Autodesk Inventor part; units mm, degrees
ref_plane "YZ Plane" through (0, 0, 0) normal (1, 0, 0) x (0, 1, 0)
ref_plane "XZ Plane" through (0, 0, 0) normal (0, 1, 0) x (-1, 0, 0)
ref_plane "XY Plane" through (0, 0, 0) normal (0, 0, 1) x (1, 0, 0)
sketch "Эскиз1" plane through (0, 0, 0) normal (0, 0, 1) x (1, 0, 0)
  line L0 (-11.75, -4.5) -> (11.75, -4.5)
  line L1 (11.75, -4.5) -> (11.75, 4.5)
  line L2 (11.75, 4.5) -> (-11.75, 4.5)
  line L3 (-11.75, 4.5) -> (-11.75, -4.5)
  line L4 (-11.75, -4.5) -> (11.75, 4.5) construction
  line L5 (11.75, -4.5) -> (-11.75, 4.5) construction
  point P0 (0, 0)
  dimension "d0" = 23.5
  dimension "d1" = 9
extrude "Выдавливание1" add sketch "Эскиз1" along normal mid plane 17
sketch "Эскиз2" plane through (0, 0, 0) normal (0, 1, 0) x (-1, 0, 0)
  line L0 (14.5, -3.1) -> (-14.5, -3.1)
  line L1 (-14.5, -3.1) -> (-14.5, -7.1)
  line L2 (-14.5, -7.1) -> (14.5, -7.1)
  line L3 (14.5, -7.1) -> (14.5, -3.1)
  line L4 (-11.75, 8.5) -> (11.75, 8.5)
  line L5 (0, 8.5) -> (0, -8.5)
  line L6 (11.75, -8.5) -> (-11.75, -8.5)
  line L7 (14.5, -5.1) -> (-14.5, -5.1)
  line L8 (13.25, -5.1) -> (-13.25, -5.1)
  circle A0 centre (13.25, -5.1) radius 0.75
  circle A1 centre (-13.25, -5.1) radius 0.75
  point P0 (0, 0)
  point P1 (0, -7.1)
  point P2 (0, -5.1)
  dimension "d4" = 29
  dimension "d5" = 4
  dimension "d6" = 26.5
  dimension "d7" = 1.5
  dimension "d8" = 1.5
  dimension "d9" = 3.4
extrude "Выдавливание2" add sketch "Эскиз2" along normal mid plane 0.95 contours L3 L7 A0 L5 L0 | L5 L7 A1 L1 L0 | L3 L2 L5 L7 A0 | L5 L2 L1 L7 A1
fillet "Сопряжение1" radius 4.5 4 edges at (-11.75, -4.5, 0) (-11.75, 4.5, 0) (11.75, 4.5, 0) (11.75, -4.5, 0)
sketch "Эскиз3" plane through (0, 0, 8.5) normal (0, 0, 1) x (1, 0, 0)
  arc A0 (7.25, -4.5) -> (7.25, 4.5) centre (7.25, 0) ccw
  circle A1 centre (7.25, 0) radius 3.5
  point P0 (0, 0)
  dimension "d13" = 7
extrude "Выдавливание3" add sketch "Эскиз3" along normal blind 3.5
sketch "Эскиз4" plane through (-7.25, 4.5, -8.5) normal (0, 1, 0) x (1, 0, 0)
  line L0 (0, -17) -> (-4.5, -17)
  line L1 (-4.5, -17) -> (-4.5, -15.5)
  line L2 (-4.5, 0) -> (-4.5, -17)
  line L3 (-4.5, -17) -> (-0.5, -17)
  line L4 (-0.5, -17) -> (-4.5, -15.5)
  point P0 (7.25, -8.5)
  dimension "d16" = 1.5
  dimension "d17" = 4
extrude "Выдавливание4" cut sketch "Эскиз4" against normal blind 20
sketch "Эскиз5" plane through (0, 0, -8.5) normal (0, 0, -1) x (-1, 0, 0)
  line L0 (14.5, -0.475) -> (14.5, 0.475)
  line L1 (14.5, 0) -> (-14.5, 0)
  line L2 (-14.5, -0.475) -> (-14.5, 0.475)
  circle A0 centre (5.95, 0) radius 4
  line L3 (12.5, 0.475) -> (12.5, -0.475)
  line L4 (12.5, 0) -> (14, 0)
  line L5 (14, 0.475) -> (14, -0.475)
  line L6 (13.25, 0) -> (5.95, 0)
  point P0 (0, 0)
  dimension "d20" = 8
  dimension "d21" = 7.3
extrude "Выдавливание5" add sketch "Эскиз5" along normal blind 0.8
sketch "Эскиз6" plane through (-5.95, 0, -9.3) normal (0, 0, -1) x (-1, 0, 0)
  circle A0 centre (0, 0) radius 1.925
  point P0 (-5.95, 0)
  dimension "d24" = 3.85
extrude "Выдавливание6" add sketch "Эскиз6" along normal blind 3
chamfer "Фаска1" distance 0.3 angle 45 1 edges at (-4.025, 0, -12.3)
sketch "Эскиз7" plane through (0, 0, -8.5) normal (0, 0, -1) x (-1, 0, 0)
  circle A0 centre (5.95, 0) radius 4
  arc A1 (-7.25, 4.5) -> (-7.25, -4.5) centre (-7.25, 0) ccw
  line L0 (-7.25, -4.5) -> (7.25, -4.5)
  arc A2 (7.25, -4.5) -> (7.25, 4.5) centre (7.25, 0) ccw
  line L1 (7.25, 4.5) -> (-7.25, 4.5)
  line L2 (7.25, -4.5) -> (-7.25, -4.5)
  line L3 (-7.25, -4.5) -> (-7.25, 4.5)
  line L4 (-7.25, 4.5) -> (7.25, 4.5)
  line L5 (7.25, 4.5) -> (7.25, -4.5)
  circle A3 centre (5.95, 0) radius 1.925
  circle A4 centre (5.95, 0) radius 4
  circle A5 centre (5.95, 0) radius 1.625
  point P0 (0, 0)
properties part number "OCS-D008 B"
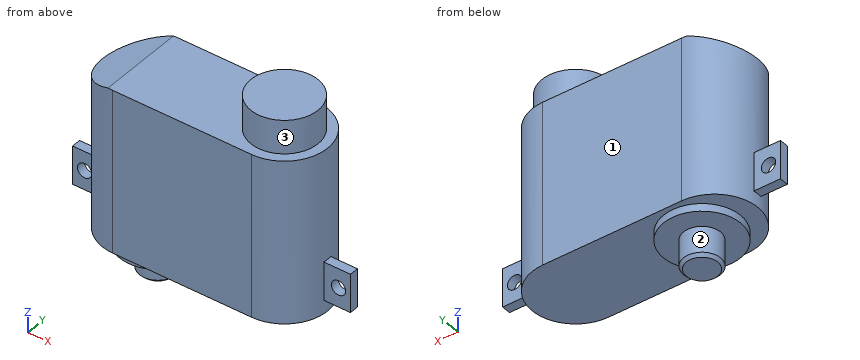
Input: part model. Units: mm. Frame: model coordinates. Face numbers are marked on the shaded views. A direction names the side the tool comes from. Give positions to 0.01 mm unless a question says otherwise; leave off trailing zeros. Order: outer loops, then holes, each group sorted by start corner. A loop starts at its lowest first (then second) coordinate and runs counter-clockwise, first axis right, second up. Notation, with made-up numbers: M 15.25,30 L 28.25,30 A22 ccw 28.25,60 Z; hole C 86.25,2 d11. An arc over 180 degrees is marked long. Return JSON: item names as keys, results as strings.
1) Access query for the marked faces 1, 2 and 3. Directions: +Z, -Z, +X, -X, +Y, -Y. A direction counts if a zero-diameter tool reaches every point of the face in a straight line with its end or side. Return the directions, or none.
Taken from the geometry:
{"face 1": "+Z, -Z, +X, -X, +Y", "face 2": "-Z", "face 3": "+Z"}
2) Line query: L1, parallel to X at y = -0.2, z = -5.1; L2, parallel to Z at x = -13.25, y = 0.1; L3, parallel to Z at x = 5.75, y = -2.75. Output: solid intervals per line, ascending. Write a range as [from, to].
Taken from the geometry:
{"L1": "x = [-14.5, -14], [-12.5, 12.5], [14, 14.5]", "L2": "z = [-7.1, -5.85], [-4.35, -3.1]", "L3": "z = [-8.5, 12]"}
3) Section query B-B on x = -5.95. Output: boundary loops of the cut face in (y, z) (3 decimals), and give its area (3 significant figures).
Taken from the geometry:
{"outline": "M -4.5,-8.5 L -4,-8.5 L -4,-9.3 L -1.925,-9.3 L -1.925,-12 L -1.625,-12.3 L 1.625,-12.3 L 1.925,-12 L 1.925,-9.3 L 4,-9.3 L 4,-8.5 L 4.5,-8.5 L 4.5,8.5 L -4.5,8.5 Z", "area": "171 mm2"}
4) Section query A-A on z = -5.1. Output: boundary loops of the cut face in (x, y) (3 decimals), and give its area (3 significant figures).
Taken from the geometry:
{"outline": "M -14.5,-0.475 L -14,-0.475 L -14,0.475 L -14.5,0.475 Z; M -12.5,-0.475 L -11.725,-0.475 A4.5 ccw -7.25,-4.5 L 7.25,-4.5 A4.5 ccw 11.725,-0.475 L 12.5,-0.475 L 12.5,0.475 L 11.725,0.475 A4.5 ccw 7.25,4.5 L -7.25,4.5 A4.5 ccw -11.725,0.475 L -12.5,0.475 Z; M 14,-0.475 L 14.5,-0.475 L 14.5,0.475 L 14,0.475 Z", "area": "197 mm2"}
5) Section query C-C on y = 2.5. Output: boundary loops of the cut face in (x, z), and give its area (3 significant figures).
Taken from the geometry:
{"outline": "M -10.99,-8.5 L -9.07,-8.5 L -9.07,-9.3 L -2.83,-9.3 L -2.83,-8.5 L 10.99,-8.5 L 10.99,8.5 L 9.7,8.5 L 9.7,12 L 4.8,12 L 4.8,8.5 L -7.75,8.5 L -10.99,7.28 Z", "area": "394 mm2"}
6) Section query D-D on z = 4. Output: boundary loops of the cut face in (x, y).
Taken from the geometry:
{"outline": "M -7.25,-4.5 L 7.25,-4.5 A4.5 ccw 7.25,4.5 L -7.25,4.5 A4.5 ccw Z"}
7) Contact query for flat-ended pins moving along their axis: pin 1 (1.4 mm diameter, centred on x = 12.5, z = -6, fed in from +Y) (3 decimals); pin 2 (4 mm diameter, centred on x = -4, y = 0.5, fed in from +Z); pin 3 (1.5 mm diameter, centred on y = -2, z = -8.5, fed in from -X). Output: stop coordinate, or through.
Taken from the geometry:
{"pin 1": "stops at y = 0.475", "pin 2": "stops at z = 8.5", "pin 3": "stops at x = -11.57"}
